Check sheet for the modelled part. Datum: model origin and axes. Units: mm. Face numbers are marked on the shaded views. A direction names the side the tool comes from. Give positions to 0.01 mm unless a question says otherwise; leave off trailing zeros. Loops run counter-clockwise (first coordinate to the right, second up) from the corner with the lowest first, then second, coordinate; pieces in that order, holes last. Notation, with made-up numbers: (33.25, 1) - (80.25, 1) arc R16 ccw to (80.25, 22) - close; hole circle Ø5 at (83.25, -14.5). An arc over 180 degrees is marked (long way). Answer in a Markdown table with one row per item. Add a question column.
(1) Draft check along X on the marked faces 1, 2 and 3. Enter one of: released by +X, released by -X, zero draft, split by the parting line, or undercut.
(2) Sectioned sample at B-B on z = 32. Enter the section's corners in (x, y).
(3) Set-up check for the marked faces 4, 5 and 6: record each of +Z, -Z, +X, -X, +Y, -Y from which the full face is reachable in a straight line by a thin tool's end or side.
(4) Sectioned sample at D-D on x = -69. Enter the section's corners in (y, z), then the cut area to 3 significant figures.
(5) Sectioned sample at A-A on z = 17.5. Enter the section's corners in (x, y).
(6) Sectioned sample at C-C on y = 3. Enter the section's corners in (x, z), then the cut area to 3 significant figures.
(7) Thickness scan on L1, parallel to Z at x = -80.5, y = 9.5; L2, parallel to X at y = -8.5, z = 28.5; L3, parallel to Y at x = -108.5, z = 13.5. Record the ranges inside material, lowest first.
(8) Go/stop test with flat-tipped pins: P1, Ø4, axis at y = 18.5, z = 24, coming from the -X side; P2, Ø1, axis at y = -5.5, z = 21.5, coming from the +X side; P3, Ø17.5, axis at x = -63, z = 15.5, coming from the +Y side. Record where each tip stops, or that it passes through.
from build123d import *

# Parameters (mm, degrees)
BOSS_EXTRUDE1_DEPTH = 35
BOSS_EXTRUDE2_DEPTH = 5
BOSS_EXTRUDE3_START = 35
BOSS_EXTRUDE3_DEPTH = 5
CUT_EXTRUDE1_DEPTH  = 137.38179019
CHAMFER1_SIZE       = 5
FILLET1_R           = 15


with BuildPart() as part:
    # Sketch1 → Boss-Extrude1 (new body)
    with BuildSketch(Plane.XY):
        Polygon((-41.540540541, -20.232432432), (-122.540540541, -20.232432432), (-122.540540541, -1.432432432), (-97.540540541, -1.432432432), (-97.540540541, 48.567567568), (-93.540540541, 48.567567568), (-93.540540541, -10.232432432), (-41.540540541, -10.232432432), align=None)
    extrude(amount=BOSS_EXTRUDE1_DEPTH)

    # Sketch3 → Boss-Extrude2 (add)
    with BuildSketch(Plane.XY):
        Polygon((-93.540540541, 24.767567568), (-93.540540541, -10.232432432), (-58.540540541, -10.232432432), align=None)
    extrude(amount=BOSS_EXTRUDE2_DEPTH)

    # Sketch3<2> → Boss-Extrude3 (add)
    with BuildSketch(Plane.XY.offset(BOSS_EXTRUDE3_START)):
        Polygon((-93.540540541, 24.767567568), (-93.540540541, -10.232432432), (-58.540540541, -10.232432432), align=None)
    extrude(amount=-BOSS_EXTRUDE3_DEPTH)

    # Sketch2 → Cut-Extrude1 (cut, through all)
    with BuildSketch(Plane(origin=(0, 0, 0), x_dir=(1, 0, 0), z_dir=(0, 1, 0))):
        with BuildLine():
            Line((-85.540540541, -12.5), (-77.540540541, -12.5))
            ThreePointArc((-77.540540541, -12.5), (-72.540540541, -17.5), (-77.540540541, -22.5))
            Line((-77.540540541, -22.5), (-85.540540541, -22.5))
            ThreePointArc((-85.540540541, -22.5), (-90.540540541, -17.5), (-85.540540541, -12.5))
        make_face()
        with BuildLine():
            Line((-60.540540541, -12.5), (-52.540540541, -12.5))
            ThreePointArc((-52.540540541, -12.5), (-47.540540541, -17.5), (-52.540540541, -22.5))
            Line((-52.540540541, -22.5), (-60.540540541, -22.5))
            ThreePointArc((-60.540540541, -22.5), (-65.540540541, -17.5), (-60.540540541, -12.5))
        make_face()
    extrude(amount=-CUT_EXTRUDE1_DEPTH, mode=Mode.SUBTRACT)

    # Chamfer1
    chamfer1_edges = [part.edges().sort_by_distance(p)[0] for p in [
        (-122.540540541, -20.232432432, 17.5),
    ]]
    chamfer(chamfer1_edges, length=CHAMFER1_SIZE)

    # Fillet1
    fillet1_edges = [part.edges().sort_by_distance(p)[0] for p in [
        (-41.540540541, -15.232432432, 0),
        (-41.540540541, -15.232432432, 35),
    ]]
    fillet(fillet1_edges, radius=FILLET1_R)


solid = part.part
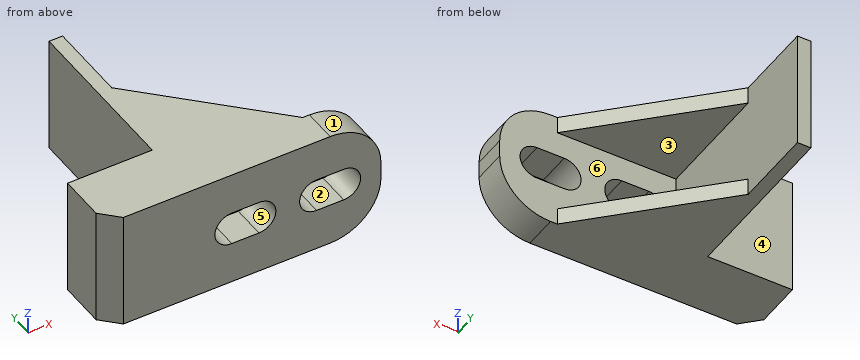
Reply:
| question | item | result |
|---|---|---|
| 1 | face 1 | released by +X |
| 1 | face 2 | undercut |
| 1 | face 3 | zero draft |
| 2 | outline | (-122.54, -15.23) - (-117.54, -20.23) - (-47.54, -20.23) - (-47.54, -10.23) - (-58.54, -10.23) - (-93.54, 24.77) - (-93.54, 48.57) - (-97.54, 48.57) - (-97.54, -1.43) - (-122.54, -1.43) - close |
| 3 | face 4 | +Z, -Z, -X, +Y |
| 3 | face 5 | +Y, -Y |
| 3 | face 6 | +X, +Y |
| 4 | outline | (-20.23, 0) - (0.23, 0) - (0.23, 5) - (-10.23, 5) - (-10.23, 30) - (0.23, 30) - (0.23, 35) - (-20.23, 35) - close |
| 4 | area | 455 mm^2 |
| 5 | outline | (-122.54, -15.23) - (-117.54, -20.23) - (-90.54, -20.23) - (-90.54, -10.23) - (-93.54, -10.23) - (-93.54, 48.57) - (-97.54, 48.57) - (-97.54, -1.43) - (-122.54, -1.43) - close; (-72.54, -20.23) - (-65.54, -20.23) - (-65.54, -10.23) - (-72.54, -10.23) - close; (-47.54, -20.23) - (-41.54, -20.23) - (-41.54, -10.23) - (-47.54, -10.23) - close |
| 6 | outline | (-97.54, 0) - (-71.77, 0) - (-71.77, 5) - (-93.54, 5) - (-93.54, 30) - (-71.77, 30) - (-71.77, 35) - (-97.54, 35) - close |
| 6 | area | 358 mm^2 |
| 7 | L1 | 0 to 5, 30 to 35 |
| 7 | L2 | -122.54 to -93.54 |
| 7 | L3 | -20.23 to -1.43 |
| 8 | P1 | x = -97.54 |
| 8 | P2 | x = -93.54 |
| 8 | P3 | y = -10.23 |
